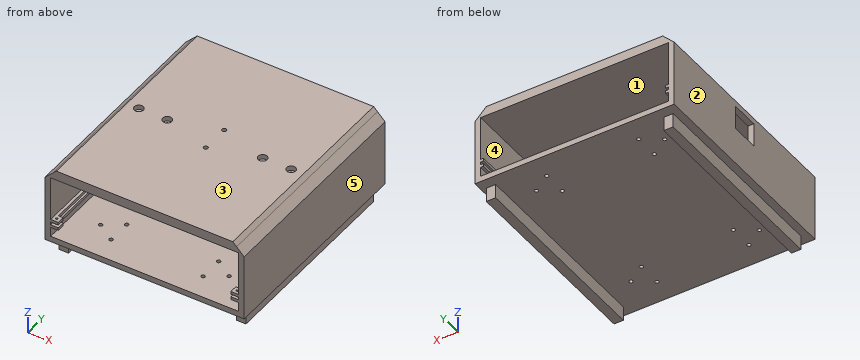
```python
from build123d import *

# Parameters (mm, degrees)
SKETCH_1_W           = 210
SKETCH_1_H           = 230
EXTRUDE_1_DEPTH      = 6
SKETCH_2_W           = 9.85
SKETCH_2_H           = 208.5
EXTRUDE_3_DEPTH      = 15
SKETCH_3_R           = 2
CUT_EXTRUDE_1_DEPTH  = 10
SKETCH_17_W          = 6
SKETCH_17_H          = 230
EXTRUDE_9_DEPTH      = 66
EXTRUDE_10_DEPTH     = 6
CHAMFER_3_SIZE       = 8
SKETCH_21_R          = 2.3
CUT_EXTRUDE_9_DEPTH  = 6
SKETCH_34_R          = 2.25
CUT_EXTRUDE_14_DEPTH = 30
SKETCH_36_R          = 2.25
CUT_EXTRUDE_15_DEPTH = 30
SKETCH_51_W          = 194
SKETCH_51_H          = 230
EXTRUDE_22_DEPTH     = 4
CHAMFER_6_SIZE       = 4
CUT_EXTRUDE_START    = -5
SKETCH_54_R          = 4.75
SKETCH_54_R_2        = 2.3
CUT_EXTRUDE_21_DEPTH = 5
CUT_EXTRUDE_23_REACH = 324.062
SKETCH_60_W          = 25
SKETCH_60_H          = 30
SKETCH_61_W          = 3
SKETCH_61_H          = 3
EXTRUDE_25_DEPTH     = 230
SKETCH_63_W          = 5
SKETCH_63_H          = 8
EXTRUDE_26_DEPTH     = 3
SKETCH_65_W          = 5
SKETCH_65_H          = 8
EXTRUDE_27_DEPTH     = 3
SKETCH_64_R          = 1.15
CUT_EXTRUDE_24_DEPTH = 9
SKETCH_66_W          = 5
SKETCH_66_H          = 8
EXTRUDE_28_DEPTH     = 3
SKETCH_67_W          = 5
SKETCH_67_H          = 8
EXTRUDE_29_DEPTH     = 3
SKETCH_68_R          = 1.15
CUT_EXTRUDE_25_DEPTH = 9


with BuildPart() as part:
    # 草图1 → 凸台-拉伸1 (new body)
    with BuildSketch(Plane.XY):
        with Locations((105, 115)):
            Rectangle(SKETCH_1_W, SKETCH_1_H)
    extrude(amount=EXTRUDE_1_DEPTH)

    # 草图2 → 凸台-拉伸3 (add)
    with BuildSketch(Plane(origin=(0, 0, 0), x_dir=(-1, 0, 0), z_dir=(0, 0, -1))):
        with Locations((-200, 115)):
            Rectangle(SKETCH_2_W, SKETCH_2_H)
        with Locations((-13, 115)):
            Rectangle(SKETCH_2_W, SKETCH_2_H)
    extrude(amount=EXTRUDE_3_DEPTH)

    # 草图3 → 切除-拉伸1 (cut)
    with BuildSketch(Plane(origin=(0, 0, 0), x_dir=(-1, 0, 0), z_dir=(0, 0, -1))):
        with Locations((-169.6425573, 192.25)):
            Circle(SKETCH_3_R)
        with Locations((-150.5, 205)):
            Circle(SKETCH_3_R)
        with Locations((-150.5, 179.5)):
            Circle(SKETCH_3_R)
        with Locations(Location((-150.5, 50.5, 0), (0, 0, 180))):
            Circle(SKETCH_3_R)
        with Locations(Location((-150.5, 25, 0), (0, 0, 180))):
            Circle(SKETCH_3_R)
        with Locations(Location((-169.6425573, 37.75, 0), (0, 0, 180))):
            Circle(SKETCH_3_R)
        with Locations((-34.3574427, 192.25)):
            Circle(SKETCH_3_R)
        with Locations((-53.5, 205)):
            Circle(SKETCH_3_R)
        with Locations((-53.5, 179.5)):
            Circle(SKETCH_3_R)
        with Locations(Location((-53.5, 50.5, 0), (0, 0, 180))):
            Circle(SKETCH_3_R)
        with Locations(Location((-53.5, 25, 0), (0, 0, 180))):
            Circle(SKETCH_3_R)
        with Locations(Location((-34.3574427, 37.75, 0), (0, 0, 180))):
            Circle(SKETCH_3_R)
    extrude(amount=-CUT_EXTRUDE_1_DEPTH, mode=Mode.SUBTRACT)

    # 草图17 → 凸台-拉伸9 (add)
    with BuildSketch(Plane.XY.offset(6)):
        with Locations((3, 115)):
            Rectangle(SKETCH_17_W, SKETCH_17_H)
        with Locations((207, 115)):
            Rectangle(SKETCH_17_W, SKETCH_17_H)
    extrude(amount=EXTRUDE_9_DEPTH)

    # 草图18 → 凸台-拉伸10 (add)
    with BuildSketch(Plane.XY.offset(72)):
        Polygon((210, 230), (204, 230), (6, 230), (0, 230), (0, 0), (6, 0), (204, 0), (210, 0), align=None)
    extrude(amount=EXTRUDE_10_DEPTH)

    # 倒角3
    chamfer_3_edges = [part.edges().sort_by_distance(p)[0] for p in [
        (210, 115, 78),
        (0, 115, 78),
    ]]
    chamfer(chamfer_3_edges, length=CHAMFER_3_SIZE)

    # 草图21 → 切除-拉伸9 (cut)
    with BuildSketch(Plane.XY.offset(72)):
        with Locations((105, 130)):
            Circle(SKETCH_21_R)
        with Locations((105, 100)):
            Circle(SKETCH_21_R)
    extrude(amount=CUT_EXTRUDE_9_DEPTH, mode=Mode.SUBTRACT)

    # 草图34 → 切除-拉伸14 (cut)
    with BuildSketch(Plane(origin=(0, 0, 72), x_dir=(-1, 0, 0), z_dir=(0, 0, -1))):
        with Locations((-185.25, 115)):
            Circle(SKETCH_34_R)
        with Locations((-155.25, 115)):
            Circle(SKETCH_34_R)
    extrude(amount=-CUT_EXTRUDE_14_DEPTH, mode=Mode.SUBTRACT)

    # 草图36 → 切除-拉伸15 (cut)
    with BuildSketch(Plane(origin=(0, 0, 72), x_dir=(-1, 0, 0), z_dir=(0, 0, -1))):
        with Locations((-54.75, 115)):
            Circle(SKETCH_36_R)
        with Locations((-24.75, 115)):
            Circle(SKETCH_36_R)
    extrude(amount=-CUT_EXTRUDE_15_DEPTH, mode=Mode.SUBTRACT)

    # 草图51 → 凸台-拉伸22 (add)
    with BuildSketch(Plane.XY.offset(78)):
        with Locations((105, 115)):
            Rectangle(SKETCH_51_W, SKETCH_51_H)
    extrude(amount=EXTRUDE_22_DEPTH)

    # 倒角6
    chamfer_6_edges = [part.edges().sort_by_distance(p)[0] for p in [
        (202, 115, 82),
        (8, 115, 82),
    ]]
    chamfer(chamfer_6_edges, length=CHAMFER_6_SIZE - 0.0001)  # a hair under: the kernel refuses the full size

    # 草图54 → 切除-拉伸21 (cut)
    with BuildSketch(Plane.XY.offset(82).offset(CUT_EXTRUDE_START)):
        with Locations((54.75, 115)):
            Circle(SKETCH_54_R)
        with Locations((105, 130)):
            Circle(SKETCH_54_R_2)
        with Locations((105, 100)):
            Circle(SKETCH_54_R_2)
        with Locations((24.75, 115)):
            Circle(SKETCH_54_R)
        with Locations((155.25, 115)):
            Circle(SKETCH_54_R)
        with Locations((185.25, 115)):
            Circle(SKETCH_54_R)
    extrude(amount=CUT_EXTRUDE_21_DEPTH, mode=Mode.SUBTRACT)

    # 草图60 → 切除-拉伸23 (cut, up to next)
    with BuildSketch(Plane.ZY, mode=Mode.PRIVATE) as cut_extrude_23_sk1:
        with Locations((51.5, 115)):
            Rectangle(SKETCH_60_W, SKETCH_60_H)
    cut_extrude_23_tool1 = extrude(cut_extrude_23_sk1.sketch, amount=-CUT_EXTRUDE_23_REACH, mode=Mode.PRIVATE) & part.part
    add(cut_extrude_23_tool1.solids().sort_by_distance((0, 115, 51.5))[0], mode=Mode.SUBTRACT)

    # 草图61 → 凸台-拉伸25 (add)
    with BuildSketch(Plane.XZ):
        with Locations((7.5, 23.5)):
            Rectangle(SKETCH_61_W, SKETCH_61_H)
        with Locations((7.5, 17.5)):
            Rectangle(SKETCH_61_W, SKETCH_61_H)
        with Locations((202.5, 17.5)):
            Rectangle(SKETCH_61_W, SKETCH_61_H)
        with Locations((202.5, 23.5)):
            Rectangle(SKETCH_61_W, SKETCH_61_H)
    extrude(amount=-EXTRUDE_25_DEPTH)

    # 草图63 → 凸台-拉伸26 (add)
    with BuildSketch(Plane.XY.offset(25)):
        with Locations((11.5, 4)):
            Rectangle(SKETCH_63_W, SKETCH_63_H)
    extrude(amount=-EXTRUDE_26_DEPTH)

    # 草图65 → 凸台-拉伸27 (add)
    with BuildSketch(Plane.XY.offset(19)):
        with Locations((11.5, 4)):
            Rectangle(SKETCH_65_W, SKETCH_65_H)
    extrude(amount=-EXTRUDE_27_DEPTH)

    # 草图64 → 切除-拉伸24 (cut)
    with BuildSketch(Plane.XY.offset(25)):
        with Locations((10, 4)):
            Circle(SKETCH_64_R)
    extrude(amount=-CUT_EXTRUDE_24_DEPTH, mode=Mode.SUBTRACT)

    # 草图66 → 凸台-拉伸28 (add)
    with BuildSketch(Plane.XY.offset(25)):
        with Locations((198.5, 4)):
            Rectangle(SKETCH_66_W, SKETCH_66_H)
    extrude(amount=-EXTRUDE_28_DEPTH)

    # 草图67 → 凸台-拉伸29 (add)
    with BuildSketch(Plane.XY.offset(19)):
        with Locations((198.5, 4)):
            Rectangle(SKETCH_67_W, SKETCH_67_H)
    extrude(amount=-EXTRUDE_29_DEPTH)

    # 草图68 → 切除-拉伸25 (cut)
    with BuildSketch(Plane.XY.offset(25)):
        with Locations((200, 4)):
            Circle(SKETCH_68_R)
    extrude(amount=-CUT_EXTRUDE_25_DEPTH, mode=Mode.SUBTRACT)


solid = part.part
```
CAD build for the part. Positions are in the model's coordinates, mm. Face numbers are marked on the shaded views. A direction names the side the tool comes from. Give positions to 0.01 mm unless a question says otherwise; leave off trailing zeros. Loops run counter-clockwise (first coordinate to the right, second up) from the corner with the lowest first, then second, coordinate; pieces in that order, holes last. Notation, with made-up numbers: (-29.5, 42) -> (15.5, 42) arc R23 ccw to (15.5, 57) -> close; hole circle Ø6 at (46, 59.25). An arc over 180 degrees is marked (long way). Use a Markdown table: item, result.
1. Flat gauge pins, fed straight in: pin 1 (10 mm diameter, centred on x = 109, y = 117, fed in from -Z); pin 2 (3.5 mm diameter, centred on x = 185.25, y = 115, fed in from +Z); pin 3 (3 mm diameter, centred on x = 3.5, y = 119.5, fed in from +Z). Where does each tip first touch, or does it go through?
Check result:
| item | result |
|---|---|
| pin 1 | stops at z = 0 |
| pin 2 | stops at z = 6 |
| pin 3 | stops at z = 75 |
2. Which spindle directions (+Z, -Z, +X, -X, +Y, -Y) get a long thin tool onto all of the face, cutting with end or side? Do the marked faces 1 and 2. Say none if no direction does.
Check result:
| item | result |
|---|---|
| face 1 | +Y, -Y |
| face 2 | +Z, -Z, -X, +Y, -Y |
3. Mould opens along Z. For the marked faces 3, 4 and 5 say: pulls with the +Z half, pulls with the -Z half, needs draft (parallel to the pull), parting line crosses it, or undercut.
Check result:
| item | result |
|---|---|
| face 3 | pulls with the +Z half |
| face 4 | undercut |
| face 5 | needs draft |
4. Wall check: L1, parallel to X at y = 206.5, z = 40; L2, parallel to Z at x = 38, y = 59; L3, parallel to Y at x = 200, z = 23. Give the ranges that are in metal, low to high. Write a range as [from, to].
Check result:
| item | result |
|---|---|
| L1 | x = [0, 6], [204, 210] |
| L2 | z = [0, 6], [72, 82] |
| L3 | y = [0, 2.85], [5.15, 8] |
5. Slice it at A-A (z = -5). List the corners of the cut face in (x, y) (3 decimals).
Check result:
| item | result |
|---|---|
| outline | (8.075, 10.75) -> (17.925, 10.75) -> (17.925, 219.25) -> (8.075, 219.25) -> close; (195.075, 10.75) -> (204.925, 10.75) -> (204.925, 219.25) -> (195.075, 219.25) -> close |
